Build history of the part. All positions in model axes, mm. Give positions to 0.01 mm unless a question says otherwise; leave off trailing zeros. Write each loop counter-clockwise with the first axis right and the second up, starting at its lowest first coordinate (ties: lowest second). Pieces come first, ordered by that corner, then holes. Notation, with made-up numbers: (59.5, 16) -> (110.5, 16) arc R25 cw to (110.5, 31) -> close; hole circle Ø11 at (45.25, 4). An arc over 180 degrees is marked (long way). Put each result on its own line as item: value.
from build123d import *

# Parameters (mm, degrees)
SKETCH_1_R               = 80
SKETCH_1_R_2             = 1.6
EXTRUDE_1_DEPTH          = 4
CUT_EXTRUDE_1_DEPTH      = 114.207773585
CUT_EXTRUDE_1_DEPTH_BACK = 114.207773585
SKETCH_2_R               = 1.6
CUT_EXTRUDE_2_DEPTH      = 114.207773585
CUT_EXTRUDE_2_DEPTH_BACK = 114.207773585
SKETCH_3_R               = 20


with BuildPart() as part:
    # 草图1 → 凸台-拉伸1 (new body)
    with BuildSketch(Plane(origin=(0, 0, 0), x_dir=(1, 0, 0), z_dir=(0, 1, 0))):
        with Locations(Location((0, 0, 0), (0, 0, 270))):
            Circle(SKETCH_1_R)
        with Locations(Location((4.784441198, 69.836302325, 0), (0, 0, 270))):
            Circle(SKETCH_1_R_2, mode=Mode.SUBTRACT)
        with Locations(Location((-62.872232519, -30.774703542, 0), (0, 0, 270))):
            Circle(SKETCH_1_R_2, mode=Mode.SUBTRACT)
        with Locations(Location((58.087791321, -39.061598783, 0), (0, 0, 270))):
            Circle(SKETCH_1_R_2, mode=Mode.SUBTRACT)
    extrude(amount=EXTRUDE_1_DEPTH)

    # 草图2 → 切除-拉伸1 (cut, two sides: drawn at the far end of the back side and taken through both)
    with BuildSketch(Plane(origin=(0, 4, 0), x_dir=(1, 0, 0), z_dir=(0, 1, 0)).offset(-CUT_EXTRUDE_1_DEPTH_BACK)):
        with Locations(Location((-62.451230924, -12.202314724, 0), (0, 0, 270))):
            Circle(SKETCH_2_R)
        with Locations(Location((62.455127781, 12.259932826, 0), (0, 0, 270))):
            Circle(SKETCH_2_R)
    extrude(amount=CUT_EXTRUDE_1_DEPTH + CUT_EXTRUDE_1_DEPTH_BACK, mode=Mode.SUBTRACT)

    # 草图3 → 切除-拉伸2 (cut, two sides: drawn at the far end of the back side and taken through both)
    with BuildSketch(Plane(origin=(0, 4, 0), x_dir=(1, 0, 0), z_dir=(0, 1, 0)).offset(-CUT_EXTRUDE_2_DEPTH_BACK)):
        with Locations(Location((0, 0, 0), (0, 0, 270))):
            Circle(SKETCH_3_R)
    extrude(amount=CUT_EXTRUDE_2_DEPTH + CUT_EXTRUDE_2_DEPTH_BACK, mode=Mode.SUBTRACT)


solid = part.part
1) Pin check, flat tips, straight feed: pin 1 (1.5 mm diameter, centred on y = 3, z = 2, fed in from -X); pin 2 (3 mm diameter, centred on x = 4.78, z = -69.84, fed in from -Y); pin 3 (1.5 mm diameter, centred on x = -41.5, y = 3.5, fed in from -Z). Stop position of each tip, or through.
Filled sheet:
pin 1: x = -79.99
pin 2: through
pin 3: z = -68.84
2) Slice it at A-A (x = 0). Write the cut outline in (y, z).
Filled sheet:
outline: (0, -80) -> (4, -80) -> (4, -20) -> (0, -20) -> close; (0, 20) -> (4, 20) -> (4, 80) -> (0, 80) -> close
3) Slice it at C-C (y = 3.2). Write the cut outline in (x, z).
Filled sheet:
outline: circle Ø160 at (0, 0); hole circle Ø3.2 at (-62.87, 30.77); hole circle Ø3.2 at (-62.45, 12.2); hole circle Ø40 at (0, 0); hole circle Ø3.2 at (4.78, -69.84); hole circle Ø3.2 at (58.09, 39.06); hole circle Ø3.2 at (62.46, -12.26)
4) Pull direction Z, two halves, no side cores. Call faces 1 (the flat face through (-17, 4, 17)), 2 (the cylindrical face through (-78.1, 1.97, -17.34)), 3 (the cylindrical face through (-19.524, 1.972, -4.336)): released by +Z, released by -Z, zero draft, split by the parting line, or undercut.
Filled sheet:
face 1: zero draft
face 2: split by the parting line
face 3: undercut
5) Slice it at D-D (z = 58). Write the cut outline in (x, y), plus the area to 3 significant figures.
Filled sheet:
outline: (-55.1, 0) -> (55.1, 0) -> (55.1, 4) -> (-55.1, 4) -> close
area: 441 mm2
6) Slice it at B-B (z = 0). Write the cut outline in (x, y).
Filled sheet:
outline: (-80, 0) -> (-20, 0) -> (-20, 4) -> (-80, 4) -> close; (20, 0) -> (80, 0) -> (80, 4) -> (20, 4) -> close
7) Wall check: L1, parallel to X at y = 2.85, z = 0; L2, parallel to X at y = 1.75, z = 12.5; L3, parallel to Z at x = -8.5, y = 2.4. Give the ranges that are in metal, low to high.
Filled sheet:
L1: -80 to -20, 20 to 80
L2: -79.02 to -64.02, -60.88 to -15.61, 15.61 to 79.02
L3: -79.55 to -18.1, 18.1 to 79.55
